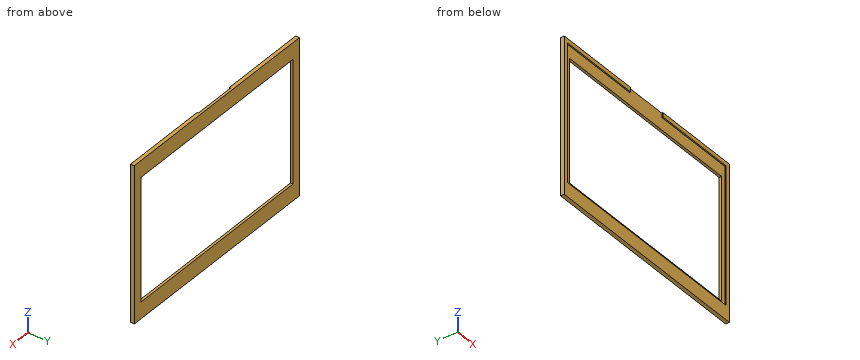
from build123d import *

# Parameters (mm, degrees)
SKETCH1_W           = 179
SKETCH1_H           = 127
SKETCH1_W_2         = 165
SKETCH1_H_2         = 100
BOSS_EXTRUDE1_DEPTH = 3
SKETCH1_3_W         = 172
SKETCH1_3_H         = 112
SKETCH1_3_W_2       = 35
SKETCH1_3_H_2       = 3.5
CUT_EXTRUDE1_DEPTH  = 1


with BuildPart() as part:
    # Sketch1 → Boss-Extrude1 (new body)
    with BuildSketch(Plane(origin=(0, 0, 0), x_dir=(1, 0, 0), z_dir=(0, 1, 0))):
        with Locations((89.5, 63.5)):
            Rectangle(SKETCH1_W, SKETCH1_H)
        with Locations((89.5, 63.5)):
            Rectangle(SKETCH1_W_2, SKETCH1_H_2, mode=Mode.SUBTRACT)
    extrude(amount=BOSS_EXTRUDE1_DEPTH)

    # Sketch1<3> → Cut-Extrude1 (cut)
    with BuildSketch(Plane(origin=(0, 0, 0), x_dir=(1, 0, 0), z_dir=(0, 1, 0))):
        with Locations((89.5, 59.5)):
            Rectangle(SKETCH1_3_W, SKETCH1_3_H)
        with Locations((89.5, 1.75)):
            Rectangle(SKETCH1_3_W_2, SKETCH1_3_H_2)
    extrude(amount=CUT_EXTRUDE1_DEPTH, mode=Mode.SUBTRACT)


solid = part.part
Work out the finished part from the listing and answer in its coordinate system (mm). Give positions to 0.01 mm unless a question says otherwise; leave off trailing zeros. Loops run counter-clockwise (first coordinate to the right, second up) from the corner with the lowest first, then second, coordinate; pieces in that order, holes last. Notation, with made-up numbers: (-32.75, -28.75) -> (25.25, -28.75) arc R8 ccw to (25.25, -24.75) -> close; hole circle Ø6 at (54.25, 11.25). An arc over 180 degrees is marked (long way). Use a Markdown table: item, result. Add a question column.
1) The part is cut by section D-D, the plane x = 58. Determine the outline of the cut face in (y, z), plus the area to 3 significant figures.
2) Consider line 1 along Z through (x, y) = (90.5, 2.45); line 2 along X through (y, z) = (2.75, -101.5); line 3 along Z through (x, y) = (49, 0.9). Determine where each line is inside the solid, lowest interval first.
3) The part is cut by section A-A, the plane x = 91. Determine the outline of the cut face in (y, z), plus the area to 3 significant figures.
4) This flat-tipped pin is pushed along its axis until it touches: P1, Ø1.1, axis at y = 0.5, z = -2, coming from the -X side. Where does it stop, or does it pass through?
5) The part is cut by section C-C, the plane y = 2.35. Determine the outline of the cut face in (x, z).
6) The part is cut by section B-B, the plane z = -59. Determine the outline of the cut face in (x, y).
Reported:
| question | item | result |
|---|---|---|
| 1 | outline | (0, -127) -> (3, -127) -> (3, -113.5) -> (1, -113.5) -> (1, -115.5) -> (0, -115.5) -> close; (0, -3.5) -> (1, -3.5) -> (1, -13.5) -> (3, -13.5) -> (3, 0) -> (0, 0) -> close |
| 1 | area | 69.0 mm^2 |
| 2 | line 1 | z = -127 to -113.5, -13.5 to 0 |
| 2 | line 2 | x = 0 to 7, 172 to 179 |
| 2 | line 3 | z = -127 to -115.5, -3.5 to 0 |
| 3 | outline | (0, -127) -> (3, -127) -> (3, -113.5) -> (1, -113.5) -> (1, -115.5) -> (0, -115.5) -> close; (1, -13.5) -> (3, -13.5) -> (3, 0) -> (1, 0) -> close |
| 3 | area | 65.5 mm^2 |
| 4 | P1 | stops at x = 0 |
| 5 | outline | (0, -127) -> (179, -127) -> (179, 0) -> (0, 0) -> close; hole (7, -113.5) -> (172, -113.5) -> (172, -13.5) -> (7, -13.5) -> close |
| 6 | outline | (0, 0) -> (3.5, 0) -> (3.5, 1) -> (7, 1) -> (7, 3) -> (0, 3) -> close; (172, 1) -> (175.5, 1) -> (175.5, 0) -> (179, 0) -> (179, 3) -> (172, 3) -> close |
